The listing builds one solid part. Answer for the finished solid, in the listing's coordinates (mm). A direction names the side the tool comes from. Give positions to 0.01 mm unless a question says otherwise; leave off trailing zeros. Write each loop counter-clockwise with the first axis right and the second up, starting at its lowest first coordinate (ties: lowest second). Pieces come first, ordered by that corner, then holes. Notation, with made-up numbers: M 82.25,34.5 L 126.25,34.5 A19 cw 126.25,60.5 Z; hole C 32,55.5 d6. An arc over 180 degrees is marked long. Answer as a JSON object with one key per item and string values.
```python
from build123d import *

# Parameters (mm, degrees)
CYLINDER006_R          = 2.4
CYLINDER006_DEPTH      = 7
CYLINDER004_R          = 4
CYLINDER004_DEPTH      = 12
CYLINDER007_R          = 2.4
CYLINDER007_DEPTH      = 7
CYLINDER005_R          = 4
CYLINDER005_DEPTH      = 12
CYLINDER_R             = 2.67
CYLINDER_DEPTH         = 2
CYLINDER001_R          = 2.67
CYLINDER001_DEPTH      = 2
CYLINDER002_R          = 2.67
CYLINDER002_DEPTH      = 2
PAD005_DEPTH           = 2
PAD006_DEPTH           = 2
PAD007_DEPTH           = 2
PAD008_DEPTH           = 2
PAD009_DEPTH           = 2
PAD010_DEPTH           = 2
PAD011_DEPTH           = 2
PAD013_DEPTH           = 2
PAD014_DEPTH           = 2
PAD015_DEPTH           = 2
PAD001_DEPTH           = 2
PAD004_DEPTH           = 2
PAD_DEPTH              = 2
CUT014_PLACEMENT_ANGLE = 180
CYLINDER003_R          = 4
CYLINDER003_DEPTH      = 12
CYLINDER008_R          = 2.4
CYLINDER008_DEPTH      = 7


with BuildPart() as cylindre006:
    # Cylinder006 → Cylinder006 (new body)
    with BuildSketch(Plane.XY.offset(10)):
        Circle(CYLINDER006_R)
    extrude(amount=CYLINDER006_DEPTH)


with BuildPart() as obj1:
    # Cylinder004 → Cylinder004 (new body)
    with BuildSketch(Plane.XY):
        Circle(CYLINDER004_R)
    extrude(amount=CYLINDER004_DEPTH)

    # Fusion001: union Cylindre006
    add(cylindre006.part)


with BuildPart() as obj1_1:
    # Fusion001 placement: moved
    add(obj1.part.moved(Location((57, -123, 0))))


with BuildPart() as cylindre007:
    # Cylinder007 → Cylinder007 (new body)
    with BuildSketch(Plane.XY.offset(10)):
        Circle(CYLINDER007_R)
    extrude(amount=CYLINDER007_DEPTH)


with BuildPart() as obj2:
    # Cylinder005 → Cylinder005 (new body)
    with BuildSketch(Plane.XY):
        Circle(CYLINDER005_R)
    extrude(amount=CYLINDER005_DEPTH)

    # Fusion002: union Cylindre007
    add(cylindre007.part)


with BuildPart() as obj2_1:
    # Fusion002 placement: moved
    add(obj2.part.moved(Location((0, -1.5, 0))))


with BuildPart() as obj3:
    # Cylinder → Cylinder (new body)
    with BuildSketch(Plane(origin=(0, -20, 0), x_dir=(1, 0, 0), z_dir=(0, 0, 1))):
        Circle(CYLINDER_R)
    extrude(amount=CYLINDER_DEPTH)


with BuildPart() as obj4:
    # Cylinder001 → Cylinder001 (new body)
    with BuildSketch(Plane(origin=(-37, -99, 0), x_dir=(1, 0, 0), z_dir=(0, 0, 1))):
        Circle(CYLINDER001_R)
    extrude(amount=CYLINDER001_DEPTH)


with BuildPart() as obj5:
    # Cylinder002 → Cylinder002 (new body)
    with BuildSketch(Plane(origin=(37, -99, 0), x_dir=(1, 0, 0), z_dir=(0, 0, 1))):
        Circle(CYLINDER002_R)
    extrude(amount=CYLINDER002_DEPTH)


with BuildPart() as pad005:
    # Sketch003 → Pad005 (new body)
    with BuildSketch(Plane(origin=(11, -73, 0), x_dir=(1, 0, 0), z_dir=(0, 0, 1))):
        with BuildLine():
            ThreePointArc((-16.037963, 9.653341), (-11.364469, 14.54891), (-16.07126, 19.412473))
            Line((-16.07126, 19.412473), (-16.07126, 17.849285))
            ThreePointArc((-16.099219, 11.213839), (-12.926154, 14.518251), (-16.07126, 17.849285))
            Line((-16.099219, 11.213839), (-16.037963, 9.653341))
        make_face()
    extrude(amount=PAD005_DEPTH)


with BuildPart() as pad006:
    # Sketch004 → Pad006 (new body)
    with BuildSketch(Plane(origin=(50, -28, 0), x_dir=(1, 0, 0), z_dir=(0, 0, 1))):
        Polygon((-60.172302, -40.014927), (-55.94516, -45.234154), (-55.94516, -50.065174), (-54.392334, -50.065174), (-54.392334, -45.234154), (-50.035789, -40.058064), (-51.804287, -40.014927), (-55.211884, -43.767593), (-58.360672, -40.014927), align=None)
    extrude(amount=PAD006_DEPTH)


with BuildPart() as pad007:
    # Sketch005 → Pad007 (new body)
    with BuildSketch(Plane(origin=(51, -113, 0), x_dir=(1, 0, 0), z_dir=(0, 0, 1))):
        Polygon((-59.924492, 29.827353), (-59.924492, 20.043087), (-51.799427, 20.043087), (-51.778122, 21.388154), (-58.539266, 21.388154), (-58.539266, 24.241791), (-54.392208, 24.241791), (-54.368668, 25.648745), (-58.563912, 25.648742), (-58.563912, 28.444752), (-51.871914, 28.444752), (-51.871914, 29.842251), align=None)
    extrude(amount=PAD007_DEPTH)


with BuildPart() as pad008:
    # Sketch006 → Pad008 (new body)
    with BuildSketch(Plane(origin=(40, -88, 0), x_dir=(1, 0, 0), z_dir=(0, 0, 1))):
        with BuildLine():
            ThreePointArc((-49.406039, -14.877108), (-44.91958, -18.684082), (-40.264656, -15.085049))
            Line((-40.264656, -10.039436), (-40.264656, -15.085049))
            Line((-41.877358, -10.014557), (-40.264656, -10.039436))
            Line((-41.877358, -14.88168), (-41.877358, -10.014557))
            ThreePointArc((-47.799763, -14.688175), (-44.913294, -17.072215), (-41.877358, -14.88168))
            Line((-47.799763, -10.014557), (-47.799763, -14.688175))
            Line((-49.406039, -10.014557), (-47.799763, -10.014557))
            Line((-49.406039, -14.877108), (-49.406039, -10.014557))
        make_face()
    extrude(amount=PAD008_DEPTH)


with BuildPart() as pad009:
    # Sketch007 → Pad009 (new body)
    with BuildSketch(Plane(origin=(40, -100, 0), x_dir=(1, 0, 0), z_dir=(0, 0, 1))):
        Polygon((-50.044407, -10.111172), (-48.184219, -10.111172), (-45.103821, -13.769145), (-41.913406, -10.083668), (-40.145214, -10.083668), (-44.168697, -14.869287), (-39.989098, -20.012453), (-41.77589, -20.012453), (-45.048813, -16.051941), (-48.266731, -20.012453), (-50.136971, -20.012453), (-46.03894, -14.924294), align=None)
    extrude(amount=PAD009_DEPTH)


with BuildPart() as pad010:
    # Sketch008 → Pad010 (new body)
    with BuildSketch(Plane(origin=(-50, -55, 0), x_dir=(1, 0, 0), z_dir=(0, 0, 1))):
        Polygon((59.944996, -10.081698), (59.944996, -20.096376), (62.215767, -20.096376), (62.215767, -14.04099), (67.572456, -20.038153), (69.901451, -20.038153), (69.901451, -9.965249), (67.397781, -9.965249), (67.397781, -16.195311), (62.099316, -10.139923), (60.294342, -10.023474), align=None)
    extrude(amount=PAD010_DEPTH)


with BuildPart() as pad011:
    # Sketch009 → Pad011 (new body)
    with BuildSketch(Plane(origin=(-50, -49, 0), x_dir=(1, 0, 0), z_dir=(0, 0, 1))):
        with BuildLine():
            ThreePointArc((69.990994, -35.138157), (65.066559, -30.24793), (60.081311, -35.076147))
            Line((60.081311, -35.076147), (62.25066, -35.155739))
            ThreePointArc((67.819598, -35.120229), (65.017788, -32.418467), (62.25066, -35.155739))
            Line((67.819598, -35.120229), (69.990994, -35.138157))
        make_face()
    extrude(amount=PAD011_DEPTH)


with BuildPart() as pad013:
    # Sketch010 → Pad013 (new body)
    with BuildSketch(Plane(origin=(-50, -50, 0), x_dir=(1, 0, 0), z_dir=(0, 0, 1))):
        with BuildLine():
            ThreePointArc((60.168351, -35.543583), (65.118967, -40.276993), (70.083354, -35.558027))
            Line((67.844375, -35.426405), (70.083354, -35.558027))
            ThreePointArc((62.41541, -35.543583), (65.184903, -38.033705), (67.844375, -35.426405))
            Line((60.168351, -35.543583), (62.41541, -35.543583))
        make_face()
    extrude(amount=PAD013_DEPTH)


with BuildPart() as pad014:
    # Sketch011 → Pad014 (new body)
    with BuildSketch(Plane(origin=(-49, -45, 0), x_dir=(1, 0, 0), z_dir=(0, 0, 1))):
        Polygon((60.004894, -50.040436), (60.004894, -60.12682), (68.854347, -60.12682), (68.854347, -58.239292), (62.037025, -58.239292), (62.037025, -55.989849), (65.320709, -55.989849), (65.320709, -54.042088), (62.078052, -54.042088), (62.078052, -52.009895), (68.356964, -52.009895), (68.356964, -50.040436), align=None)
    extrude(amount=PAD014_DEPTH)


with BuildPart() as pad015:
    # Sketch012 → Pad015 (new body)
    with BuildSketch(Plane(origin=(-59, -10, 0), x_dir=(1, 0, 0), z_dir=(0, 0, 1))):
        Polygon((70.077477, -99.382187), (70.077477, -110.073188), (77.927521, -110.073188), (77.927521, -108.204124), (72.395118, -108.204124), (72.395118, -99.382187), align=None)
    extrude(amount=PAD015_DEPTH)


with BuildPart() as pad001:
    # Sketch001 → Pad001 (new body)
    with BuildSketch(Plane(origin=(24, -79, 0), x_dir=(1, 0, 0), z_dir=(0, 0, 1))):
        Polygon((-31.011786, 39.876404), (-25.943949, 39.876404), (-25.943949, 38.661366), (-26.762781, 38.678547), (-26.762781, 29.865536), (-33.84618, 29.865536), (-33.84618, 31.212646), (-28.189131, 31.212646), (-28.189131, 38.604298), (-31.618616, 38.604298), (-31.618616, 39.928497), align=None)
    extrude(amount=PAD001_DEPTH)


with BuildPart() as pad004:
    # Sketch002 → Pad004 (new body)
    with BuildSketch(Plane(origin=(23, -75, 0), x_dir=(1, 0, 0), z_dir=(0, 0, 1))):
        with BuildLine():
            ThreePointArc((-29.06636, 21.208672), (-33.855078, 16.402926), (-29.050702, 11.612834))
            Line((-29.040989, 13.272719), (-29.050702, 11.612834))
            ThreePointArc((-28.975843, 19.558972), (-32.109932, 16.447987), (-29.040989, 13.272719))
            Line((-29.06636, 21.208672), (-28.975843, 19.558972))
        make_face()
    extrude(amount=PAD004_DEPTH)


with BuildPart() as cut014:
    # Sketch → Pad (new body)
    with BuildSketch(Plane(origin=(0, 0, 0), x_dir=(0, 1, 0), z_dir=(0, 0, 1))):
        Polygon((-130.055618, 74.700851), (-130.055618, -75.434654), (-99.793674, -44.971566), (-99.793674, -60.477265), (-69.960533, -30.215105), (-69.960533, -45.106522), (-39.827045, -19.776331), (-39.827045, -34.952637), (10.030094, 0.023063), (-39.838676, 35.327641), (-39.838676, 19.908756), (-70.002281, 44.561149), (-70.002281, 28.932402), (-100.276372, 60.120483), (-100.276372, 44.971665), align=None)
    extrude(amount=PAD_DEPTH)

    # Cut001: cut Pad004
    add(pad004.part, mode=Mode.SUBTRACT)

    # Cut: cut Pad001
    add(pad001.part, mode=Mode.SUBTRACT)

    # Cut002: cut Pad015
    add(pad015.part, mode=Mode.SUBTRACT)

    # Cut003: cut Pad014
    add(pad014.part, mode=Mode.SUBTRACT)

    # Cut004: cut Pad013
    add(pad013.part, mode=Mode.SUBTRACT)

    # Cut005: cut Pad011
    add(pad011.part, mode=Mode.SUBTRACT)

    # Cut006: cut Pad010
    add(pad010.part, mode=Mode.SUBTRACT)

    # Cut007: cut Pad009
    add(pad009.part, mode=Mode.SUBTRACT)

    # Cut008: cut Pad008
    add(pad008.part, mode=Mode.SUBTRACT)

    # Cut009: cut Pad007
    add(pad007.part, mode=Mode.SUBTRACT)

    # Cut010: cut Pad006
    add(pad006.part, mode=Mode.SUBTRACT)

    # Cut011: cut Pad005
    add(pad005.part, mode=Mode.SUBTRACT)

    # Cut012: cut obj5
    add(obj5.part, mode=Mode.SUBTRACT)

    # Cut013: cut obj4
    add(obj4.part, mode=Mode.SUBTRACT)

    # Cut014: cut obj3
    add(obj3.part, mode=Mode.SUBTRACT)


with BuildPart() as cut014_1:
    # Cut014 placement: moved
    add(cut014.part.rotate(Axis((0, 0, 0), (0, 1, 0)), CUT014_PLACEMENT_ANGLE))


with BuildPart() as cylindre003:
    # Cylinder003 → Cylinder003 (new body)
    with BuildSketch(Plane.XY):
        Circle(CYLINDER003_R)
    extrude(amount=CYLINDER003_DEPTH)


with BuildPart() as fusion005:
    # Cylinder008 → Cylinder008 (new body)
    with BuildSketch(Plane.XY.offset(10)):
        Circle(CYLINDER008_R)
    extrude(amount=CYLINDER008_DEPTH)

    # Fusion: union Cylindre003
    add(cylindre003.part)


with BuildPart() as fusion005_1:
    # Fusion placement: moved
    add(fusion005.part.moved(Location((-57, -123, 0))))

    # Fusion003: union Cut014
    add(cut014_1.part)

    # Fusion004: union obj2
    add(obj2_1.part)

    # Fusion005: union obj1
    add(obj1_1.part)


solid = fusion005_1.part
```
1. A cutting plane is placed at C-C, the plane x = 37. Give the vertices of the cut face in (y, z).
Verdict:
{"outline": "M -130.06,-2 L -101.67,-2 L -101.67,0 L -130.06,0 Z; M -96.33,-2 L -77.83,-2 L -77.83,0 L -96.33,0 Z; M -70,-2 L -60.75,-2 L -60.75,0 L -70,0 Z"}
2. Flat-ended cylindrical pins translate along their axes: pin 1 (0.6 mm diameter, centred on y = -104.5, z = -1, fed in from +X); pin 2 (1.1 mm diameter, centred on y = -48.5, z = -1, fed in from -X); pin 3 (3 mm diameter, centred on x = -6.5, z = 7, fed in from -Y); pin 4 (2 mm diameter, centred on x = 0.5, z = -1.5, fed in from +Y). Find the tip coordinate at first contact, or state that the pin passes through.
Verdict:
{"pin 1": "stops at x = 49.49", "pin 2": "stops at x = -27.53", "pin 3": "passes through", "pin 4": "stops at y = 10.03"}
3. A cutting plane is placed at B-B, the plane z = 2.5. Give the vertices of the cut face in (x, y), plus the area to 3 significant figures.
Verdict:
{"outline": "C -57,-123 d8; C 0,-1.5 d8; C 57,-123 d8", "area": "151 mm2"}
4. A cutting plane is placed at D-D, the plane z = 13.75. Give the vertices of the cut face in (x, y).
Verdict:
{"outline": "C -57,-123 d4.8; C 0,-1.5 d4.8; C 57,-123 d4.8"}
5. For faces 1 (the flat face through (-14.86, -72, -0.99)), 2 (the flat face through (44.31, -84.93, -0.99)), 3 (the flat face through (-57, -123, 17)), 4 (the flat face through (-45.56, -85.09, -0.99)), 5 (the cylindrical face through (-57.31, -120.62, 14.46)), determine the directions among +Z, -Z, +X, -X, +Y, -Y from which every point of the face is accessible in a straight line to the end or side of a thin tool.
Verdict:
{"face 1": "+Z, -Z", "face 2": "+Z, -Z, +X", "face 3": "+Z, +X, -X, +Y, -Y", "face 4": "+Z, -Z, -X", "face 5": "+Z"}
6. Consider line 1 along Y through (x, z) = (37, -1.2); line 2 along Y through (x, z) = (-37, -1.3); line 3 along Z through (x, y) = (-21, -62). Determine where each line is inside the solid, lowest interval first.
Verdict:
{"line 1": "y = -130.06 to -101.67, -96.33 to -77.83, -70 to -60.75", "line 2": "y = -130.06 to -101.67, -96.33 to -76.65, -69.96 to -60.32", "line 3": "z = -2 to 0"}
7. A cutting plane is placed at A-A, the plane x = 57. Give the vertices of the cut face in (y, z), plus the area to 3 significant figures.
Verdict:
{"outline": "M -130.06,-2 L -112.32,-2 L -112.32,0 L -119,0 L -119,12 L -120.6,12 L -120.6,17 L -125.4,17 L -125.4,12 L -127,12 L -127,0 L -130.06,0 Z; M -100.28,-2 L -97.25,-2 L -97.25,0 L -100.28,0 Z", "area": "162 mm2"}
8. The mould has two halves that part along X. Classify faces 6 (the cylindrical face through (-38.23, -101.37, -0.99)), 7 (the flat face through (8.117, -117.504, -0.986)), 8 (the flat face through (1, -77, -2)), 9 (the flat face through (59.63, -114.96, -0.99)): released by +X, released by -X, zero draft, split by the parting line, or undercut.
Verdict:
{"face 6": "undercut", "face 7": "undercut", "face 8": "zero draft", "face 9": "released by +X"}
